Input: part model. Units: mm. Frame: model coordinates. Face numbers are marked on the shaded views. A direction names the side the tool comes from. Round coordinates to 2 decimals unless told otherwise and drop trailing zeros. Order: outer loops, then holes, each group sorted by start corner. A loop starts at its lowest first (then second) coordinate and runs counter-clockwise, first axis right, second up. Notation, with made-up numbers: (-20.75, 18.25) -> (22.25, 18.25) arc R22 ccw to (22.25, 37.25) -> close; hole circle Ø7 at (-25, 14). An arc over 180 degrees is marked (long way). Answer as CSV lines item,"result". Start each with the question number.
1) Section query B-B, the plane z = 43. State how many separate pieces and enclosed holes the cut face has, and give its area (3 significant figures).
2) First-contact query: P1, Ø1.2, axis at x = 164.71, y = 160, coming from the -Z side; P2, Ø4, axis at y = 148.5, z = 7.5, coming from the +X side; P3, Ø5, axis at x = 164.5, z = 18, coming from the +Y side. Flat tips, straight axial feed; report the tip coordinate or a pass-through.
3) Section query A-A, the plane x = 154. Output: boundary loops of the cut face in (y, z).
4) Access query for the marked faces 4 and 5. Directions: +Z, -Z, +X, -X, +Y, -Y. A direction counts if a zero-diameter tool reaches every point of the face in a straight line with its end or side. Return the directions, or none.
5) Line query: L1, parallel to Z at x = 153, y = 154; L2, parallel to Y at x = 171.5, z = 33.5; L3, parallel to Y at x = 172.5, z = 39. Output: solid intervals per line, ascending.
6) Mould query, pull axis X, two halves, no side actions, for the marked faces 1, 2 and 3. Classes: +X half, -X half, draft (parallel to the pull), parting line (faces both ways), or undercut.
```python
from build123d import *

# Parameters (mm, degrees)
SKETCH1_R             = 1.5
BOSS_EXTRUDE2_DEPTH   = 50
BODY_MOVE_COPY1_ANGLE = 45
SKETCH2_W             = 22
SKETCH2_H             = 41
CUT_EXTRUDE1_DEPTH    = 20
CUT_EXTRUDE6_REACH    = 248.506
SKETCH4_R             = 1
SKETCH5_R             = 2
CUT_EXTRUDE7_DEPTH    = 3.5
CUT_EXTRUDE11_REACH   = 248.506
SKETCH7_R             = 1
SKETCH8_R             = 2
CUT_EXTRUDE12_DEPTH   = 3.5
SKETCH9_R             = 1.5
CUT_EXTRUDE13_DEPTH   = 247.505542905
CUT_EXTRUDE14_DEPTH   = 247.505542905
FILLET1_R             = 5


with BuildPart() as part:
    # Sketch1 → Boss-Extrude2 (new body)
    with BuildSketch(Plane.XY):
        with BuildLine():
            Line((182.281997607, 145.957424373), (161.068794171, 167.170627808))
            ThreePointArc((161.068794171, 167.170627808), (157.547403451, 168.588083689), (154.045255639, 167.12372906))
            add(Edge.make_bspline(
                [(130.757413054, 145.551615227), (143.638496584, 155.63010859), (154.045255639, 167.12372906)],
                knots=[0.85894257, 0.85894257, 0.85894257, 1, 1, 1], degree=2))
            Line((130.757413054, 145.551615227), (160.757413054, 115.551615227))
            add(Edge.make_bspline(
                [(160.757413054, 115.551615227), (170.835906417, 128.432698758), (182.329526886, 138.839457812)],
                knots=[0.85894257, 0.85894257, 0.85894257, 1, 1, 1], degree=2))
            ThreePointArc((182.329526886, 138.839457812), (183.793881516, 142.408377812), (182.281997607, 145.957424373))
        make_face()
        with Locations((157.580789545, 163.588195154)):
            Circle(SKETCH1_R, mode=Mode.SUBTRACT)
        with Locations((178.79399298, 142.374991718)):
            Circle(SKETCH1_R, mode=Mode.SUBTRACT)
    extrude(amount=BOSS_EXTRUDE2_DEPTH)


with BuildPart() as part_1:
    # Body-Move/Copy1: moved
    add(part.part.rotate(Axis((157.275703017, 142.069905191, 0), (0, 0, 1)), BODY_MOVE_COPY1_ANGLE))

    # Sketch2 → Cut-Extrude1 (cut)
    with BuildSketch(Plane(origin=(0, 162.500916843, 0), x_dir=(1, 0, 0), z_dir=(0, 1, 0))):
        with Locations((157.208932318, -25)):
            Rectangle(SKETCH2_W, SKETCH2_H)
    extrude(amount=-CUT_EXTRUDE1_DEPTH, mode=Mode.SUBTRACT)

    # Sketch4 → Cut-Extrude6 (cut, up to next)
    with BuildSketch(Plane.XY.offset(50), mode=Mode.PRIVATE) as cut_extrude6_sk1:
        with Locations((150.208932318, 152.500916843)):
            Circle(SKETCH4_R)
    cut_extrude6_tool1 = extrude(cut_extrude6_sk1.sketch, amount=-CUT_EXTRUDE6_REACH, mode=Mode.PRIVATE) & part_1.part
    # Sketch4 → Cut-Extrude6 (cut, up to next)
    with BuildSketch(Plane.XY.offset(50), mode=Mode.PRIVATE) as cut_extrude6_sk2:
        with Locations((164.208932318, 152.500916843)):
            Circle(SKETCH4_R)
    cut_extrude6_tool2 = extrude(cut_extrude6_sk2.sketch, amount=-CUT_EXTRUDE6_REACH, mode=Mode.PRIVATE) & part_1.part
    # Sketch4 → Cut-Extrude6 (cut, up to next)
    with BuildSketch(Plane.XY.offset(50), mode=Mode.PRIVATE) as cut_extrude6_sk3:
        with Locations((157.245778438, 145.500039202)):
            Circle(SKETCH4_R)
    cut_extrude6_tool3 = extrude(cut_extrude6_sk3.sketch, amount=-CUT_EXTRUDE6_REACH, mode=Mode.PRIVATE) & part_1.part
    add(cut_extrude6_tool1.solids().sort_by_distance((150.208932, 152.500917, 50))[0], mode=Mode.SUBTRACT)
    add(cut_extrude6_tool2.solids().sort_by_distance((164.208932, 152.500917, 50))[0], mode=Mode.SUBTRACT)
    add(cut_extrude6_tool3.solids().sort_by_distance((157.245778, 145.500039, 50))[0], mode=Mode.SUBTRACT)

    # Sketch5 → Cut-Extrude7 (cut)
    with BuildSketch(Plane.XY.offset(50)):
        with Locations((150.208932318, 152.500916843)):
            Circle(SKETCH5_R)
        with Locations((164.208932318, 152.500916843)):
            Circle(SKETCH5_R)
        with Locations((157.245778438, 145.500039202)):
            Circle(SKETCH5_R)
    extrude(amount=-CUT_EXTRUDE7_DEPTH, mode=Mode.SUBTRACT)

    # Sketch7 → Cut-Extrude11 (cut, up to next)
    with BuildSketch(Plane(origin=(0, 0, 0), x_dir=(-1, 0, 0), z_dir=(0, 0, -1)), mode=Mode.PRIVATE) as cut_extrude11_sk1:
        with Locations((-149.708932317, 160.000916845)):
            Circle(SKETCH7_R)
    cut_extrude11_tool1 = extrude(cut_extrude11_sk1.sketch, amount=-CUT_EXTRUDE11_REACH, mode=Mode.PRIVATE) & part_1.part
    # Sketch7 → Cut-Extrude11 (cut, up to next)
    with BuildSketch(Plane(origin=(0, 0, 0), x_dir=(-1, 0, 0), z_dir=(0, 0, -1)), mode=Mode.PRIVATE) as cut_extrude11_sk2:
        with Locations((-164.70893232, 160.000916845)):
            Circle(SKETCH7_R)
    cut_extrude11_tool2 = extrude(cut_extrude11_sk2.sketch, amount=-CUT_EXTRUDE11_REACH, mode=Mode.PRIVATE) & part_1.part
    # Sketch7 → Cut-Extrude11 (cut, up to next)
    with BuildSketch(Plane(origin=(0, 0, 0), x_dir=(-1, 0, 0), z_dir=(0, 0, -1)), mode=Mode.PRIVATE) as cut_extrude11_sk3:
        with Locations((-149.708932317, 145.000916842)):
            Circle(SKETCH7_R)
    cut_extrude11_tool3 = extrude(cut_extrude11_sk3.sketch, amount=-CUT_EXTRUDE11_REACH, mode=Mode.PRIVATE) & part_1.part
    # Sketch7 → Cut-Extrude11 (cut, up to next)
    with BuildSketch(Plane(origin=(0, 0, 0), x_dir=(-1, 0, 0), z_dir=(0, 0, -1)), mode=Mode.PRIVATE) as cut_extrude11_sk4:
        with Locations((-164.70893232, 145.000916842)):
            Circle(SKETCH7_R)
    cut_extrude11_tool4 = extrude(cut_extrude11_sk4.sketch, amount=-CUT_EXTRUDE11_REACH, mode=Mode.PRIVATE) & part_1.part
    add(cut_extrude11_tool1.solids().sort_by_distance((149.708932, 160.000917, 0))[0], mode=Mode.SUBTRACT)
    add(cut_extrude11_tool2.solids().sort_by_distance((164.708932, 160.000917, 0))[0], mode=Mode.SUBTRACT)
    add(cut_extrude11_tool3.solids().sort_by_distance((149.708932, 145.000917, 0))[0], mode=Mode.SUBTRACT)
    add(cut_extrude11_tool4.solids().sort_by_distance((164.708932, 145.000917, 0))[0], mode=Mode.SUBTRACT)

    # Sketch8 → Cut-Extrude12 (cut)
    with BuildSketch(Plane(origin=(0, 0, 0), x_dir=(-1, 0, 0), z_dir=(0, 0, -1))):
        with Locations((-164.70893232, 160.000916845)):
            Circle(SKETCH8_R)
        with Locations((-149.708932317, 160.000916845)):
            Circle(SKETCH8_R)
        with Locations((-149.708932317, 145.000916842)):
            Circle(SKETCH8_R)
        with Locations((-164.70893232, 145.000916842)):
            Circle(SKETCH8_R)
    extrude(amount=-CUT_EXTRUDE12_DEPTH, mode=Mode.SUBTRACT)

    # Sketch9 → Cut-Extrude13 (cut, through all)
    with BuildSketch(Plane(origin=(0, 0, 0), x_dir=(-1, 0, 0), z_dir=(0, 0, -1))):
        with Locations((-172.275703017, 137.501362696)):
            Circle(SKETCH9_R)
        with Locations((-142.275703017, 137.501362696)):
            Circle(SKETCH9_R)
    extrude(amount=-CUT_EXTRUDE13_DEPTH, mode=Mode.SUBTRACT)

    # Sketch10 → Cut-Extrude14 (cut, through all)
    with BuildSketch(Plane(origin=(0, 0, 0), x_dir=(-1, 0, 0), z_dir=(0, 0, -1))):
        with BuildLine():
            Line((-136.767866361, 132.501362696), (-177.783539673, 132.501362696))
            add(Edge.make_bspline(
                [(-177.783539673, 132.501362696), (-178.076738818, 129.157172087), (-178.488906453, 125.780583309)],
                knots=[0.970662354, 0.970662354, 0.970662354, 1, 1, 1], degree=2))
            Line((-178.488906453, 125.780583309), (-136.062499581, 125.780583309))
            add(Edge.make_bspline(
                [(-136.062499581, 125.780583309), (-136.474667216, 129.157172087), (-136.767866361, 132.501362696)],
                knots=[0.85894257, 0.85894257, 0.85894257, 0.888280216, 0.888280216, 0.888280216], degree=2))
        make_face()
    extrude(amount=-CUT_EXTRUDE14_DEPTH, mode=Mode.SUBTRACT)

    # Fillet1
    fillet1_edges = [part_1.edges().sort_by_distance(p)[0] for p in [
        (136.767866361, 132.501362696, 25),
        (177.783539673, 132.501362696, 25),
    ]]
    fillet(fillet1_edges, radius=FILLET1_R)


solid = part_1.part
```
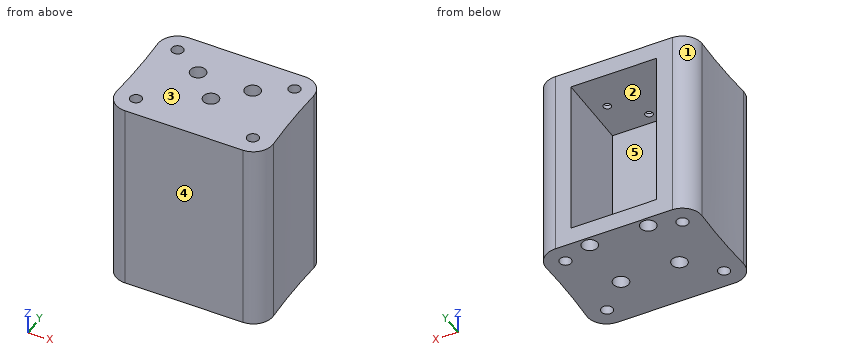
Findings:
1,separate pieces,"1"
1,enclosed holes,"4"
1,area,"707 mm^2"
2,P1,"stops at z = 45.5"
2,P2,"stops at x = 177.08"
2,P3,"stops at y = 142.5"
3,outline,"(132.5, 0) -> (162.5, 0) -> (162.5, 4.5) -> (142.5, 4.5) -> (142.5, 45.5) -> (162.5, 45.5) -> (162.5, 50) -> (132.5, 50) -> close"
4,face 4,"+Z, -Z, +X, -X, -Y"
4,face 5,"+Y"
5,L1,"z = 0 to 4.5, 45.5 to 50"
5,L2,"y = 132.5 to 136.22, 138.79 to 156.22, 158.79 to 162.5"
5,L3,"y = 132.5 to 136.02, 138.98 to 156.02, 158.98 to 162.5"
6,face 1,"-X half"
6,face 2,"undercut"
6,face 3,"draft"
